Read the model definition and answer for the solid it produces. Units are mm, in the model's axes. A direction names the side the tool comes from. Round coordinates to 2 decimals unless told otherwise and drop trailing zeros. Write each loop counter-clockwise with the first axis right and the second up, starting at its lowest first coordinate (ties: lowest second). Pieces come first, ordered by that corner, then holes. Notation, with made-up numbers: (19.5, -26) -> (31.5, -26) arc R15 cw to (31.5, -20) -> close; hole circle Ø6 at (66, 75.25). An arc over 180 degrees is marked (long way). Return JSON: item names as keys, results as strings.
Autodesk Inventor part; units mm, degrees
ref_plane "YZ Plane" through (0, 0, 0) normal (1, 0, 0) x (0, 1, 0)
ref_plane "XZ Plane" through (0, 0, 0) normal (0, 1, 0) x (-1, 0, 0)
ref_plane "XY Plane" through (0, 0, 0) normal (0, 0, 1) x (1, 0, 0)
sketch "Sketch1" plane through (0, 0, 0) normal (0, 1, 0) x (-1, 0, 0)
  line L0 (-3.0226, 8.128) -> (3.0226, 8.128)
  line L1 (3.0226, 8.128) -> (3.0226, -8.128)
  line L2 (3.0226, -8.128) -> (-3.0226, -8.128)
  line L3 (-3.0226, -8.128) -> (-3.0226, 8.128)
  line L4 (-3.0226, 8.128) -> (3.0226, -8.128) construction
  line L5 (3.0226, 8.128) -> (-3.0226, -8.128) construction
  line L6 (1.651, 0.9398) -> (1.651, -4.3454)
  line L7 (-1.651, 0.9398) -> (-1.651, -4.3454)
  arc A0 (-1.651, -4.3454) -> (1.651, -4.3454) centre (0, -4.1402) ccw
  arc A1 (1.651, 0.9398) -> (-1.651, 0.9398) centre (0, 0.9398) ccw
  line L8 (0, 9.1418) -> (0, -10.0518)
  point P0 (0, 0)
  point P1 (0, 8.128)
  dimension "d0" = 16.256
  dimension "d1" = 6.0452
  dimension "d27" = 3.302
  dimension "d28" = 1.6637
  dimension "d29" = 3.0226
  dimension "d30" = 5.08
extrude "Plate1" add sketch "Sketch1" along normal blind 1.4986 contours L0 L8 A1 L7 A0 L2 L3 | L0 L1 L2 L8 A0 L6 A1
sketch "Sketch2" plane through (3.0226, 0, 6.6294) normal (0, 0, 1) x (1, 0, 0)
  line L0 (-6.0452, 0) -> (0, 0)
  line L1 (0, 0) -> (0, 10.922)
  line L2 (0, 10.922) -> (-6.0452, 10.922)
  line L3 (-6.0452, 10.922) -> (-6.0452, 0)
edge flange "Flange1" height 10.922 angle 90 thickness 1.4986 bend radius 1.4986 thickness toward (0, 0, 1) relief straight relief width 1.4986 relief depth 0.7493 edges at (0, 1.4986, 8.128) wall of the first edge with corners at (-3.0226, 0, 6.6294) (3.0226, 0, 6.6294) (3.0226, 10.922, 6.6294) (-3.0226, 10.922, 6.6294)
bend "Bend1"
corner "Corner1"
sketch "Sketch4" plane through (3.0226, 10.922, 6.6294) normal (0, 0, -1) x (-1, 0, 0)
  circle A0 centre (3.0226, -3.683) radius 1.524
  line L0 (6.0452, 0) -> (0, 0)
  line L1 (0, -10.922) -> (6.0452, -10.922)
  point P0 (3.0226, -10.922)
  dimension "d22" = 3.048
  dimension "d25" = 7.239
extrude "Extrusion3" cut sketch "Sketch4" against normal blind 1.4986
equation "\"d11\" = BendReliefWidth"
equation "\"d12\" = BendReliefDepth"
equation "\"d13\" = MinimumRemnant"
equation "\"d14\" = BendRadius"
equation "\"d17\" = BendRadius"
equation "\"d18\" = CornerReliefSize"
equation "\"d19\" = GapSize"
equation "\"d20\" = JacobiRadiusSize"
equation "\"BendRadius\" = Thickness"
equation "\"BendReliefWidth\" = Thickness"
equation "\"BendReliefDepth\" = 0.5 * Thickness"
equation "\"CornerReliefSize\" = 4 * Thickness"
equation "\"MinimumRemnant\" = 2 * Thickness"
equation "\"TransitionRadius\" = BendRadius"
equation "\"JacobiRadiusSize\" = Thickness"
equation "\"GapSize\" = Thickness"
equation "\"d10\" = BendRadius"
properties part number "dsub37Bracket"
Item 1: Flat-ended cylindrical pins translate along their axes: pin 1 (6 mm diameter, centred on y = 6, z = -6, fed in from -X); pin 2 (2 mm diameter, centred on x = -2, y = 8.5, fed in from -Z). Find the tip coordinate at first contact, or state that the pin passes through.
Worked answers:
{"pin 1": "passes through", "pin 2": "stops at z = 6.63"}
Item 2: Section C-C (y = 6) is taken. Give the vertices of the cut face in (x, z).
Worked answers:
{"outline": "(-3.02, 6.63) -> (-0.89, 6.63) -> (-0.89, 8.13) -> (-3.02, 8.13) -> close; (0.89, 6.63) -> (3.02, 6.63) -> (3.02, 8.13) -> (0.89, 8.13) -> close"}
Item 3: Section B-B (z = 0.25) is taken. Give the vertices of the cut face in (x, y), then the cut area to 3 significant figures.
Worked answers:
{"outline": "(-3.02, 0) -> (-1.65, 0) -> (-1.65, 1.5) -> (-3.02, 1.5) -> close; (1.65, 0) -> (3.02, 0) -> (3.02, 1.5) -> (1.65, 1.5) -> close", "area": "4.11 mm2"}
Item 4: Section A-A (x = 0) is taken. Give the vertices of the cut face in (y, z) (3 decimals), then the cut area to 3 significant figures.
Worked answers:
{"outline": "(0, -8.128) -> (1.499, -8.128) -> (1.499, -5.804) -> (0, -5.804) -> close; (0, 2.591) -> (1.499, 2.591) -> (1.499, 5.131) arc R1.499 cw to (2.997, 6.629) -> (5.715, 6.629) -> (5.715, 8.128) -> (2.997, 8.128) arc R2.997 ccw to (0, 5.131) -> close; (8.763, 6.629) -> (10.922, 6.629) -> (10.922, 8.128) -> (8.763, 8.128) -> close", "area": "19.9 mm2"}
Item 5: Straight lines are drawn through the part: L1, parallel to X at y = 1, z = -3.5; L2, parallel to Z at x = 1.25, y = 6.25; L3, parallel to Y at x = 2, z = 4. For each, find the intervals that lie inside material, in ascending order. Write a range as [from, to].
Worked answers:
{"L1": "x = [-3.02, -1.65], [1.65, 3.02]", "L2": "z = [6.63, 8.13]", "L3": "y = [0, 1.5]"}
Item 6: A tool of negligible diameter and unlimited length cuts with its end or side. For faces 4 (the cylindrical face through (0.04, 0.74, 2.59)), 5 (the flat face through (2, 0, -1)), 6 (the flat face through (1.4, 6, 6.629)), from which of +Z, -Z, +X, -X, +Y, -Y can it reach the whole face along a straight path? Write none if from no direction.
Worked answers:
{"face 4": "+Y, -Y", "face 5": "+Z, -Z, +X, -X, -Y", "face 6": "-Z, +X, -X, +Y"}
Item 7: Section D-D (x = 2.25) is taken. Give the vertices of the cut face in (y, z).
Worked answers:
{"outline": "(0, -8.13) -> (1.5, -8.13) -> (1.5, 5.13) arc R1.5 cw to (3, 6.63) -> (10.92, 6.63) -> (10.92, 8.13) -> (3, 8.13) arc R3 ccw to (0, 5.13) -> close"}
Item 8: For a pull along X with two mould halves and no side action, classify faces 1 (the flat face through (3.023, 1, 4)), 2 (the flat face through (0, 1, -8.128)), 3 (the cylindrical face through (-0.034, 0.739, -5.804)) as released by +X, released by -X, zero draft, split by the parting line, or undercut.
Worked answers:
{"face 1": "released by +X", "face 2": "zero draft", "face 3": "undercut"}
